Autodesk Inventor part; units mm, degrees
ref_plane "YZ Plane" through (0, 0, 0) normal (1, 0, 0) x (0, 1, 0)
ref_plane "XZ Plane" through (0, 0, 0) normal (0, 1, 0) x (-1, 0, 0)
ref_plane "XY Plane" through (0, 0, 0) normal (0, 0, 1) x (1, 0, 0)
sketch "Sketch1" plane through (0, 0, 0) normal (0, 1, 0) x (-1, 0, 0)
  line L0 (-3.175, 0) -> (-26.035, 0)
  line L1 (-26.035, -241.3) -> (-3.175, -241.3)
  line L2 (0, -238.125) -> (0, -3.175)
  circle A0 centre (-6.35, -6.35) radius 2.2225
  circle A1 centre (-6.35, -19.05) radius 2.2225
  circle A2 centre (-6.35, -234.95) radius 2.2225
  circle A3 centre (-6.35, -222.25) radius 2.2225
  arc A4 (0, -3.175) -> (-3.175, 0) centre (-3.175, -3.175) ccw
  arc A5 (-3.175, -241.3) -> (0, -238.125) centre (-3.175, -238.125) ccw
  line L3 (-26.035, -241.3) -> (-29.21, -241.3)
  line L4 (-29.21, -241.3) -> (-33.655, -241.3)
  line L5 (-36.83, -238.125) -> (-36.83, -3.175)
  line L6 (-33.655, 0) -> (-29.21, 0)
  arc A6 (-36.83, -238.125) -> (-33.655, -241.3) centre (-33.655, -238.125) ccw
  arc A7 (-33.655, 0) -> (-36.83, -3.175) centre (-33.655, -3.175) ccw
  line L7 (-26.035, 0) -> (-31.4325, 0)
  point P0 (0, 0)
  point P1 (0, -241.3)
  point P2 (-36.83, -241.3)
  dimension "d0" = 29.21
  dimension "d2" = 4.445
  dimension "d3" = 4.445
  dimension "d4" = 4.445
  dimension "d5" = 4.445
  dimension "d6" = 3.175
  dimension "d7" = 7.62
  dimension "d8" = 3.175
  dimension "d9" = 3.175
extrude "Extrusion1" add sketch "Sketch1" along normal blind 1.778
properties part number "holder_wedge"
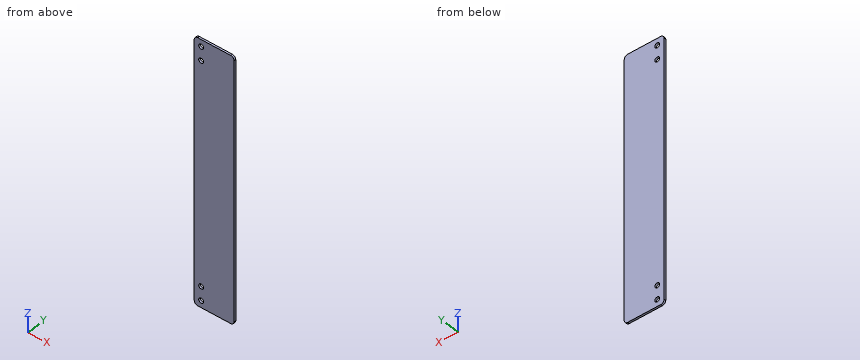
The listing builds one solid part. Answer for the finished solid, in the listing's coordinates (mm). Round coordinates to 2 decimals unless told otherwise and drop trailing zeros. Write each loop counter-clockwise with the first axis right and the second up, starting at its lowest first coordinate (ties: lowest second). Pieces come first, ordered by that corner, then holes. Notation, with made-up numbers: M 9,80.5 L 25,80.5 A25 ccw 25,111.5 Z; hole C 79,89 d1. An arc over 180 degrees is marked long. Write each question's results on one line, items separated by ' | '. Start each with the question number.
Item 1: Find section A-A on z = -234.95. Write down the section's boundary in (x, y).
Item 2: Find section B-B on x = 6.35. Write down the section's boundary in (y, z).
Item 3: Straight lines are drawn through the part: probe 1 along Z at (x, y) = (6.35, 0.75); probe 2 along X at (y, z) = (0.6, -222.25); probe 3 along Z at (x, y) = (7, 0.35). For each, find the intervals that lie inside material, in ascending order.
Answer block:
1) outline: M 0,0 L 4.13,0 L 4.13,1.78 L 0,1.78 Z; M 8.57,0 L 36.83,0 L 36.83,1.78 L 8.57,1.78 Z
2) outline: M 0,-241.3 L 1.78,-241.3 L 1.78,-237.17 L 0,-237.17 Z; M 0,-232.73 L 1.78,-232.73 L 1.78,-224.47 L 0,-224.47 Z; M 0,-220.03 L 1.78,-220.03 L 1.78,-21.27 L 0,-21.27 Z; M 0,-16.83 L 1.78,-16.83 L 1.78,-8.57 L 0,-8.57 Z; M 0,-4.13 L 1.78,-4.13 L 1.78,0 L 0,0 Z
3) probe 1: z = -241.3 to -237.17, -232.73 to -224.47, -220.03 to -21.27, -16.83 to -8.57, -4.13 to 0 | probe 2: x = 0 to 4.13, 8.57 to 36.83 | probe 3: z = -241.3 to -237.08, -232.82 to -224.38, -220.12 to -21.18, -16.92 to -8.48, -4.22 to 0
